Autodesk Inventor part; units mm, degrees
ref_plane "YZ Plane" through (0, 0, 0) normal (1, 0, 0) x (0, 1, 0)
ref_plane "XZ Plane" through (0, 0, 0) normal (0, 1, 0) x (-1, 0, 0)
ref_plane "XY Plane" through (0, 0, 0) normal (0, 0, 1) x (1, 0, 0)
sketch "Szkic1" plane through (0, 0, 0) normal (0, 1, 0) x (-1, 0, 0)
  circle A0 centre (20.670805, 15.489913) radius 2.25
  circle A1 centre (20.670805, -15.489913) radius 2.25
  line L0 (-2.43121, 25.942308) -> (-19.284188, 11.800981)
  line L1 (-19.284188, 11.800981) -> (-28.926002, 23.291647)
  line L2 (-28.802745, 24.700479) -> (-28.926002, 23.291647)
  line L3 (-28.802745, 24.700479) -> (-12.715812, 38.199019)
  line L4 (-12.715812, 38.199019) -> (-2.43121, 25.942308)
  line L5 (-26.423342, -11) -> (-26.423342, 11)
  line L6 (-26.423342, 11) -> (-10.423342, 11)
  line L7 (-10.423342, 11) -> (-10.423342, -11)
  line L8 (-10.423342, -11) -> (-26.423342, -11)
  line L9 (-19.284188, -11.800981) -> (-2.43121, -25.942308)
  line L10 (-2.43121, -25.942308) -> (-12.715812, -38.199019)
  line L11 (-12.715812, -38.199019) -> (-28.802745, -24.700479)
  line L12 (-28.926002, -23.291647) -> (-28.802745, -24.700479)
  line L13 (-28.926002, -23.291647) -> (-19.284188, -11.800981)
  arc A2 (24.913446, -19.732553) -> (26.214082, -17.786013) centre (20.670805, -15.489913) ccw
  line L14 (29.391036, -10.116167) -> (26.214082, -17.786013)
  arc A3 (29.391036, -10.116167) -> (30, -7.0547) centre (22, -7.0547) ccw
  line L15 (30, -7.0547) -> (30, 7.0547)
  arc A4 (30, 7.0547) -> (29.391036, 10.116167) centre (22, 7.0547) ccw
  line L16 (26.214082, 17.786013) -> (29.391036, 10.116167)
  arc A5 (26.214082, 17.786013) -> (24.913446, 19.732553) centre (20.670805, 15.489913) ccw
  line L17 (24.913446, 19.732553) -> (9.732553, 34.913446)
  arc A6 (9.732553, 34.913446) -> (7.786013, 36.214082) centre (5.489913, 30.670805) ccw
  line L18 (0.116167, 39.391036) -> (7.786013, 36.214082)
  arc A7 (0.116167, 39.391036) -> (-2.9453, 40) centre (-2.9453, 32) ccw
  line L19 (-2.9453, 40) -> (-18.300026, 40)
  arc A8 (-18.300026, 40) -> (-24.727902, 37.660444) centre (-18.300026, 30) ccw
  line L20 (-24.727902, 37.660444) -> (-26.427876, 36.233997)
  arc A9 (-26.427876, 36.233997) -> (-30, 28.573552) centre (-20, 28.573552) ccw
  line L21 (-30, 28.573552) -> (-30, -28.573552)
  arc A10 (-30, -28.573552) -> (-26.427876, -36.233997) centre (-20, -28.573552) ccw
  line L22 (-26.427876, -36.233997) -> (-24.727902, -37.660444)
  arc A11 (-24.727902, -37.660444) -> (-18.300026, -40) centre (-18.300026, -30) ccw
  line L23 (-18.300026, -40) -> (-2.9453, -40)
  arc A12 (-2.9453, -40) -> (0.116167, -39.391036) centre (-2.9453, -32) ccw
  line L24 (7.786013, -36.214082) -> (0.116167, -39.391036)
  arc A13 (7.786013, -36.214082) -> (9.732553, -34.913446) centre (5.489913, -30.670805) ccw
  line L25 (9.732553, -34.913446) -> (24.913446, -19.732553)
  circle A14 centre (0, -18) radius 2.25
  circle A15 centre (0, 18) radius 2.25
  ellipse E0 centre (5.489913, 0.077944) end of major axis (-3.705883, 0.077944) minor radius 9.366229
  point P0 (0, 0)
  point P1 (0, 0)
extrude "Wyciągnięcie proste1" add sketch "Szkic1" along normal blind 3 contours L0 L1 L2 L3 L4 | L5 L6 L7 L8 | L9 L10 L11 L12 L13 | L25 A13 L24 A12 L23 A11 L22 A10 L21 A9 L20 A8 L19 A7 L18 A6 L17 A5 L16 A4 L15 A3 L14 A2
chamfer "Faza1" distance 2 angle 45 1 edges at (-5.4899, 3, 9.4442)
chamfer "Faza2" distance 2 angle 45 4 edges at (-18.4208, 3, 15.4899) (2.25, 3, 18) (-18.4208, 3, -15.4899) (2.25, 3, -18)
fillet "Zaokrąglenie1" radius 3 24 edges at (30, 3, 0) (29.0631, 3, -32.7997) (25.5779, 3, -36.9472) (21.7202, 3, -39.3969) (10.6227, 3, -40) (1.3846, 3, -39.8463) (-3.9511, 3, -37.8026) (-8.8233, 3, -35.6596) (-17.323, 3, -27.323) (-25.6596, 3, -18.8233) (-27.8026, 3, -13.9511) (-29.8463, 3, -8.6154) (-30, 3, 0) (-29.8463, 3, 8.6154) (-27.8026, 3, 13.9511) (-25.6596, 3, 18.8233) (-17.323, 3, 27.323) (-8.8233, 3, 35.6596) (-3.9511, 3, 37.8026) (1.3846, 3, 39.8463) (10.6227, 3, 40) (21.7202, 3, 39.3969) (25.5779, 3, 36.9472) (29.0631, 3, 32.7997)
properties part number "obudowa do czujnikow odleglosci v3,2 - przykrywka"
Geometry: final body of the model. Coordinates: model frame, mm. Coordinates: 2 decimals unless noted, no trailing zeros. Order: outer loops, then holes, each group sorted by start corner. A loop starts at its lowest first (then second) coordinate and runs counter-clockwise, first axis right, second up. Notation, with made-up numbers: (73.5, 59.25) - (99.5, 59.25) arc R4 ccw to (99.5, 64.25) - close; hole circle Ø1 at (17, -31). An arc over 180 degrees is marked (long way). Return JSON: item names as keys, results as strings. Group by question number.
1. Cut plane B-B (x = 11). Output: boundary loops of the cut face in (y, z).
2. Pull-direction query (Z, two-part tool) for faces 1 (the face through (-18.92, 1.13, -13.88)), 2 (the face through (-20.38, 0.49, -17.72)), 3 (the face through (-26.95, 2.14, 13.66)), 4 (the face through (-3.66, 2.14, -36.95)); classes: pulls with the +Z half, pulls with the -Z half, needs draft (parallel to the pull), parting line crosses it, or undercut.
3. Material intervals for line 1 along Z through (x, y) = (1, 0.3); line 2 along Z through (x, y) = (-19.5, 0.8); line 3 along Z through (x, y) = (0, 0.4), sorted ascending. Write a range as [from, to].
4. Pin query (flat end, axial travel): pin 1 (7 mm diameter, centred on x = -20.67, z = 15.49, fed in from +Y); pin 2 (1.5 mm diameter, centred on x = 18.5, y = 1.5, fed in from -Z); pin 3 (3.5 mm diameter, centred on x = 0, z = -18, fed in from +Y); pin 4 (1 mm diameter, centred on y = 1, z = 5, fed in from +X). Return the tip coordinate at first contact, or that it passes through.
5. Cut plane A-A (x = -22). Count the separate pieces of the cut face and the enclosed holes in it, plus the area to 3 significant figures.
Resolved:
{
 "1": {"outline": "(0, -40) arc R3 ccw to (3, -37) - (3, 37) arc R3 ccw to (0, 40) - close"},
 "2": {"face 1": "undercut", "face 2": "undercut", "face 3": "pulls with the +Z half", "face 4": "pulls with the -Z half"},
 "3": {"line 1": "z = [-39.74, -20.02], [-15.98, -6.56], [6.71, 15.98], [20.02, 39.74]", "line 2": "z = [-24.99, -17.41], [-13.57, 13.57], [17.41, 24.99]", "line 3": "z = [-39.41, -20.25], [-15.75, -7.44], [7.59, 15.75], [20.25, 39.41]"},
 "4": {"pin 1": "stops at y = 2.25", "pin 2": "stops at z = -39.9", "pin 3": "passes through", "pin 4": "stops at x = 29.96"},
 "5": {"separate pieces": "3", "enclosed holes": "0", "area": "99.6 mm²"}
}
